Design review of the part built by this model. Coordinates are the model's own, in mm. A direction names the side the tool comes from. Give positions to 0.01 mm unless a question says otherwise; leave off trailing zeros. Order: outer loops, then holes, each group sorted by start corner. A loop starts at its lowest first (then second) coordinate and runs counter-clockwise, first axis right, second up.
Autodesk Inventor part; units mm, degrees
ref_plane "YZ Plane" through (0, 0, 0) normal (1, 0, 0) x (0, 1, 0)
ref_plane "XZ Plane" through (0, 0, 0) normal (0, 1, 0) x (-1, 0, 0)
ref_plane "XY Plane" through (0, 0, 0) normal (0, 0, 1) x (1, 0, 0)
sketch "Эскиз1" plane through (0, 0, 0) normal (0, 0, 1) x (1, 0, 0)
  line L0 (0, 0) -> (5.2, 0)
  line L1 (5.2, 0) -> (5.2, 6.4)
  line L2 (5.2, 6.4) -> (0, 6.4)
  line L3 (0, 6.4) -> (0, 0)
  line L4 (8.5, 0) -> (13.7, 0)
  line L5 (13.7, 0) -> (13.7, 6.4)
  line L6 (13.7, 6.4) -> (8.5, 6.4)
  line L7 (8.5, 6.4) -> (8.5, 0)
  line L8 (17, 0) -> (22.2, 0)
  line L9 (22.2, 0) -> (22.2, 6.4)
  line L10 (22.2, 6.4) -> (17, 6.4)
  line L11 (17, 6.4) -> (17, 0)
  line L12 (25.5, 0) -> (30.7, 0)
  line L13 (30.7, 0) -> (30.7, 6.4)
  line L14 (30.7, 6.4) -> (25.5, 6.4)
  line L15 (25.5, 6.4) -> (25.5, 0)
  line L16 (5.2, 6.4) -> (8.5, 6.4)
  line L17 (13.7, 6.4) -> (17, 6.4)
  line L18 (22.2, 6.4) -> (25.5, 6.4)
  line L19 (22.2, 5.2) -> (25.5, 5.2)
  line L20 (17, 5.2) -> (13.7, 5.2)
  line L21 (8.5, 5.2) -> (5.2, 5.2)
  line L22 (0, 5.2) -> (-1.6, 5.2)
  line L23 (-1.6, 5.2) -> (-1.6, 6.4)
  line L24 (-1.6, 6.4) -> (0, 6.4)
  line L25 (0, 6.4) -> (0, 5.2)
  line L26 (30.7, 5.2) -> (32.3, 5.2)
  line L27 (32.3, 5.2) -> (32.3, 6.4)
  line L28 (32.3, 6.4) -> (30.7, 6.4)
  line L29 (30.7, 6.4) -> (30.7, 5.2)
  point P0 (0, 6.4)
  dimension "d0" = 5.2
  dimension "d1" = 6.4
  dimension "d4" = 8.5
  dimension "d9" = 1.2
  dimension "d10" = 1.6
extrude "Выдавливание1" add sketch "Эскиз1" along normal blind 0.5
sketch "Эскиз2" plane through (0, 0, 0.5) normal (0, 0, 1) x (1, 0, 0)
  line L0 (0, 5.2) -> (0, 0)
  line L1 (5.2, 0) -> (5.2, 5.2)
  line L2 (0, 1) -> (5.2, 1)
  line L3 (5.2, 1) -> (5.2, 5.5)
  line L4 (5.2, 5.5) -> (0, 5.5)
  line L5 (0, 5.5) -> (0, 1)
  line L6 (8.5, 5.2) -> (8.5, 0)
  line L7 (13.7, 0) -> (13.7, 5.2)
  line L8 (8.5, 1) -> (13.7, 1)
  line L9 (13.7, 1) -> (13.7, 5.5)
  line L10 (13.7, 5.5) -> (8.5, 5.5)
  line L11 (8.5, 5.5) -> (8.5, 1)
  line L12 (17, 5.2) -> (17, 0)
  line L13 (22.2, 0) -> (22.2, 5.2)
  line L14 (17, 1) -> (22.2, 1)
  line L15 (22.2, 1) -> (22.2, 5.5)
  line L16 (22.2, 5.5) -> (17, 5.5)
  line L17 (17, 5.5) -> (17, 1)
  line L18 (25.5, 5.2) -> (25.5, 0)
  line L19 (30.7, 0) -> (30.7, 5.2)
  line L20 (25.5, 1) -> (30.7, 1)
  line L21 (30.7, 1) -> (30.7, 5.5)
  line L22 (30.7, 5.5) -> (25.5, 5.5)
  line L23 (25.5, 5.5) -> (25.5, 1)
  line L24 (0, 0) -> (5.2, 0)
  point P0 (25.5, 5)
  point P1 (17, 5)
  point P2 (8.5, 5)
  point P3 (0, 5)
  dimension "d13" = 1
  dimension "d14" = 4.5
extrude "Выдавливание2" add sketch "Эскиз2" along normal blind 2 contours L5 L4 L3 L1 L2 L0 | L11 L10 L9 L7 L8 L6 | L17 L16 L15 L13 L14 L12 | L23 L22 L21 L19 L20 L18
sketch "Эскиз3" plane through (0, 0, 0) normal (-1, 0, 0) x (0, 0, 1)
  line L0 (0.5, 1) -> (2.5, 1.25)
  line L1 (0, 5.2) -> (0, 0)
  line L2 (0, 0) -> (0.5, 0)
  line L3 (0.5, 1) -> (0.5, 0)
  line L4 (0.5, 1) -> (2.5, 1)
  line L5 (2.5, 5.5) -> (2.5, 1)
  line L6 (0.5, 5.2) -> (0.5, 5.5)
  line L7 (0, 5.2) -> (0.5, 5.2)
  line L8 (0.5, 1) -> (2.5, 1)
  line L9 (0.5, 5.5) -> (2.5, 5.5)
  line L10 (0.5, 5.5) -> (2.5, 5.25)
  line L11 (2.5, 1) -> (2.5, 5.5)
  line L12 (2.5, 1.25) -> (2.5, 1)
  line L13 (0.5, 5.5) -> (2.5, 5.5)
  line L14 (0.5, 6.4) -> (0.5, 5.2)
  line L15 (2.5, 5.5) -> (2.5, 1)
  line L16 (2.5, 5.25) -> (2.5, 5.5)
  point P0 (2, 5.8)
  point P1 (2, 5.6739)
  point P2 (2, 5.8)
  dimension "d18" = 4
extrude "Выдавливание3" cut sketch "Эскиз3" against normal through all contours L0 L5 L4 | L10 L9 L5
properties part number "Buttons"
1. Take a section at D-D (x = 22.5). State the section outline as (y, z) points, then the cut area to 3 significant figures.
Recorded:
outline: (5.2, 0) - (6.4, 0) - (6.4, 0.5) - (5.2, 0.5) - close
area: 0.600 mm2
2. Machinability: for faces 3 (the face through (19.6, 0.5, 0.5)), 4 (the face through (28.064, 5.377, 1.486)), which of the approach directions +Z, -Z, +X, -X, +Y, -Y give a long, thin tool a straight path to every point of the face, cutting with its end or side? Answer none if there is none.
Recorded:
face 3: +Z, +X, -X, -Y
face 4: +Z, +X, -X, +Y
3. For pin 1 (0.8 mm diameter, centred on x = 27, y = 0.5, fed in from +Z); pin 2 (0.8 mm diameter, centred on y = 3.5, z = 1.5, fed in from -X); pin 3 (1.5 mm diameter, centred on y = 1, z = 1, fed in from +X), all flat-tipped, find the tip position at first contact; note any pin that passes through.
Recorded:
pin 1: stops at z = 0.5
pin 2: stops at x = 0
pin 3: stops at x = 30.7
4. Take a section at C-C (x = 4). State the section outline as (y, z) points, then the cut area to 3 significant figures.
Recorded:
outline: (0, 0) - (6.4, 0) - (6.4, 0.5) - (5.5, 0.5) - (5.25, 2.5) - (1.25, 2.5) - (1, 0.5) - (0, 0.5) - close
area: 11.7 mm2
5. For line 1 along X through (y, z) = (3.25, 2); line 2 along Z through (x, y) = (24.5, 5.25); line 3 along Y through (x, z) = (4, 1.5) (3 decimals), list the stretches that pass through material, from the lowest coordinate up.
Recorded:
line 1: x = 0 to 5.2, 8.5 to 13.7, 17 to 22.2, 25.5 to 30.7
line 2: z = 0 to 0.5
line 3: y = 1.125 to 5.375
6. Draft analysis for pull direction X (two halves, no side actions). For faces 1 (the face through (11.1, 0.5, 0.5)), 2 (the face through (13.7, 3, 1)), state which applies: pulls with the +X half, pulls with the -X half, needs draft (parallel to the pull), parting line crosses it, or undercut.
Recorded:
face 1: needs draft
face 2: undercut
7. Take a section at B-B (y = 4.25). State the section outline as (x, z) points, then the cut area to 3 significant figures.
Recorded:
outline: (0, 0) - (5.2, 0) - (5.2, 2.5) - (0, 2.5) - close; (8.5, 0) - (13.7, 0) - (13.7, 2.5) - (8.5, 2.5) - close; (17, 0) - (22.2, 0) - (22.2, 2.5) - (17, 2.5) - close; (25.5, 0) - (30.7, 0) - (30.7, 2.5) - (25.5, 2.5) - close
area: 52.0 mm2
8. Take a section at A-A (z = 1.7). State the section outline as (x, y) points.
Recorded:
outline: (0, 1.15) - (5.2, 1.15) - (5.2, 5.35) - (0, 5.35) - close; (8.5, 1.15) - (13.7, 1.15) - (13.7, 5.35) - (8.5, 5.35) - close; (17, 1.15) - (22.2, 1.15) - (22.2, 5.35) - (17, 5.35) - close; (25.5, 1.15) - (30.7, 1.15) - (30.7, 5.35) - (25.5, 5.35) - close
